Autodesk Inventor part; units mm, degrees
ref_plane "YZ Plane" through (0, 0, 0) normal (1, 0, 0) x (0, 1, 0)
ref_plane "XZ Plane" through (0, 0, 0) normal (0, 1, 0) x (-1, 0, 0)
ref_plane "XY Plane" through (0, 0, 0) normal (0, 0, 1) x (1, 0, 0)
sketch "Sketch1" plane through (0, 0, 0) normal (0, 0, 1) x (1, 0, 0)
  line L0 (0, 5.4993) -> (0, 312.0007)
  line L1 (4.7625, 314.7504) -> (47.9059, 289.8415)
  line L2 (0, 158.75) -> (212.725, 158.75) construction
  line L3 (4.7625, 2.7496) -> (47.9059, 27.6585)
  line L4 (49.4934, 287.0919) -> (49.4934, 30.4081)
  arc A0 (49.4934, 287.0919) -> (47.9059, 289.8415) centre (46.3184, 287.0919) ccw
  arc A1 (47.9059, 27.6585) -> (49.4934, 30.4081) centre (46.3184, 30.4081) ccw
  arc A2 (0, 5.4993) -> (4.7625, 2.7496) centre (3.175, 5.4993) ccw
  arc A3 (4.7625, 314.7504) -> (0, 312.0007) centre (3.175, 312.0007) ccw
  point P0 (0, 0)
  point P1 (0, 317.5)
  point P2 (49.4934, 288.925)
  point P3 (49.4934, 28.575)
  dimension "d0" = 317.5
  dimension "d1" = 57.15
  dimension "d2" = 60
  dimension "d3" = 3.175
  dimension "d4" = 3.175
extrude "Extrusion1" add sketch "Sketch1" along normal blind 536.575
sketch "Sketch4" plane through (49.4934, 30.4081, 0) normal (1, 0, 0) x (0, 0, -1)
  line L0 (-536.575, 0) -> (-536.575, 256.6838) construction
  line L1 (-536.575, 128.3419) -> (0, 128.3419) construction
  line L2 (0, 0) -> (0, 256.6838) construction
  line L3 (0, 256.6838) -> (-536.575, 256.6838) construction
  line L4 (-268.2875, 256.6838) -> (-268.2875, 0) construction
  line L5 (0, 0) -> (-536.575, 0) construction
  line L6 (-328.6125, 188.6669) -> (-207.9625, 188.6669)
  line L7 (-207.9625, 188.6669) -> (-207.9625, 68.0169)
  line L8 (-207.9625, 68.0169) -> (-328.6125, 68.0169)
  line L9 (-328.6125, 68.0169) -> (-328.6125, 188.6669)
  line L10 (-328.6125, 188.6669) -> (-207.9625, 68.0169) construction
  line L11 (-207.9625, 188.6669) -> (-328.6125, 68.0169) construction
  point P0 (0, -30.4081)
  point P1 (-268.2875, 128.3419)
  dimension "d9" = 120.65
  dimension "d10" = 120.65
extrude "Extrusion2" cut sketch "Sketch4" against normal blind 19.05
sketch "Sketch5" plane through (30.4434, 30.4081, 0) normal (1, 0, 0) x (0, 0, -1)
  circle A0 centre (-218.6305, 175.9669) radius 1.5875
  circle A1 centre (-320.2305, 175.9669) radius 1.5875
  circle A2 centre (-218.6305, 74.3669) radius 1.5875
  circle A3 centre (-320.2305, 74.3669) radius 1.5875
  line L0 (-328.6125, 68.0169) -> (-328.6125, 188.6669)
  line L1 (-207.9625, 68.0169) -> (-328.6125, 68.0169)
  line L2 (-320.2305, 175.9669) -> (-218.6305, 175.9669) construction
  line L3 (-218.6305, 175.9669) -> (-218.6305, 74.3669) construction
  line L4 (-218.6305, 74.3669) -> (-320.2305, 74.3669) construction
  line L5 (-320.2305, 74.3669) -> (-320.2305, 175.9669) construction
  point P0 (0, -30.4081)
  dimension "d13" = 3.175
  dimension "d14" = 3.175
  dimension "d15" = 3.175
  dimension "d16" = 101.6
  dimension "d17" = 101.6
  dimension "d18" = 101.6
  dimension "d19" = 8.382
  dimension "d20" = 8.382
  dimension "d21" = 107.95
extrude "Extrusion3" cut sketch "Sketch5" against normal blind 12.7
sketch "Sketch6" plane through (0, 5.4993, 0) normal (-1, 0, 0) x (0, 0, 1)
  line L0 (0, 306.5015) -> (0, 0) construction
  line L1 (0, 153.2507) -> (536.575, 153.2507) construction
  line L2 (536.575, 24.9088) -> (536.575, 281.5927) construction
  line L3 (0, 309.6765) -> (536.575, 309.6765) construction
  line L4 (0, 0) -> (536.575, 0) construction
  line L5 (0, -3.175) -> (536.575, -3.175) construction
  line L6 (268.2875, -3.175) -> (268.2875, 309.6765) construction
  line L7 (11.1125, 296.1257) -> (525.4625, 296.1257)
  line L8 (525.4625, 296.1257) -> (525.4625, 10.3757)
  line L9 (525.4625, 10.3757) -> (11.1125, 10.3757)
  line L10 (11.1125, 10.3757) -> (11.1125, 296.1257)
  line L11 (11.1125, 296.1257) -> (525.4625, 10.3757) construction
  line L12 (525.4625, 296.1257) -> (11.1125, 10.3757) construction
  point P0 (0, -5.4993)
  point P1 (268.2875, 153.2507)
  dimension "d24" = 285.75
extrude "Extrusion4" cut sketch "Sketch6" against normal blind 3.175
properties part number "Monitor v1.0"
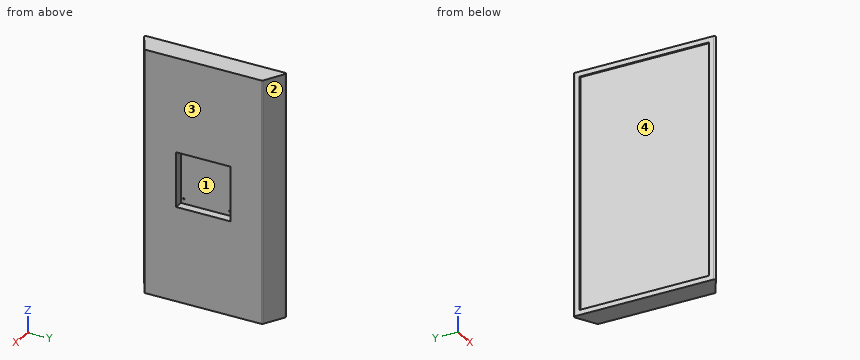
The listing builds one solid part. Answer for the finished solid, in the listing's coordinates (mm). Face numbers are marked on the shaded views. A direction names the side the tool comes from. Round coordinates to 2 decimals unless told otherwise and drop trailing zeros. Write each loop counter-clockwise with the first axis right and the second up, starting at its lowest first coordinate (ties: lowest second). Pieces come first, ordered by that corner, then holes. Notation, with made-up numbers: (74.25, 25) -> (93.25, 25) arc R13 ccw to (93.25, 31) -> close; hole circle Ø2 at (-27, -9.75). An arc over 180 degrees is marked (long way). Answer as a JSON object with one key per item and string values. Group by question number.
Q1. Determine the mould class of the marked faces 1 and 2 for opening direction Z: pulls with the +Z half, pulls with the -Z half, needs draft (parallel to the pull), parting line crosses it, or undercut.
Q2. Straight lines are drawn through the part: line 1 along Z through (x, y) = (3, 80.5) (1 decimal); line 2 along Y through (x, z) = (27.5, 437); line 3 along Z through (x, y) = (43, 150.5) (1 decimal). For each, find the intervals that lie inside material, in ascending order.
Q3. Which of the six approach directions +Z, -Z, +X, -X, +Y, -Y give full straight-line access (tool end or side, diameter ignored) to the marked faces 3 and 4?
Q4. Section B-B (y = 64) is taken. Write down the section's boundary in (x, z) (1 decimal), plus the area to 3 significant figures.
Q5. Each of these flat-tipped pins is pushed along its axis until it touches: pin 1 Ø2 at (x, z) = (29, 339) entering from -Y; pin 2 Ø3.5 at (y, z) = (206.38, 218.63) entering from +X; pin 3 Ø21 at (x, y) = (37.5, 141) entering from -Z; pin 4 Ø9.5 at (x, z) = (42.5, 250) entering from +Y (3 decimals). Where does it stop, or does it pass through?
Q6. Section D-D (y = 127) is taken. Write down the section's boundary in (x, z) (1 decimal).
Check values:
{
 "1": {"face 1": "undercut", "face 2": "needs draft"},
 "2": {"line 1": "0 to 11.1, 525.5 to 536.6", "line 2": "15.88 to 301.62", "line 3": "0 to 208, 328.6 to 536.6"},
 "3": {"face 3": "+Z, -Z, +X, +Y, -Y", "face 4": "-X"},
 "4": {"outline": "(0, 0) -> (49.5, 0) -> (49.5, 536.6) -> (0, 536.6) -> (0, 525.5) -> (3.2, 525.5) -> (3.2, 11.1) -> (0, 11.1) -> close", "area": "24,900 mm^2"},
 "5": {"pin 1": "y = 16.17", "pin 2": "x = 30.44", "pin 3": "z = 0", "pin 4": "y = 295.705"},
 "6": {"outline": "(0, 0) -> (49.5, 0) -> (49.5, 208) -> (30.4, 208) -> (30.4, 328.6) -> (49.5, 328.6) -> (49.5, 536.6) -> (0, 536.6) -> (0, 525.5) -> (3.2, 525.5) -> (3.2, 11.1) -> (0, 11.1) -> close"}
}
